Verification items for the finished model (mm, model axes). A direction names the side the tool comes from. Round coordinates to 2 decimals unless told otherwise and drop trailing zeros. Loops run counter-clockwise (first coordinate to the right, second up) from the corner with the lowest first, then second, coordinate; pieces in that order, holes last. Notation, with made-up numbers: M -23.5,-30 L 27.5,-30 A9 ccw 27.5,-13 Z; hole C 82,53.25 d9. An arc over 180 degrees is marked long. One line per item, written item: value.
from build123d import *

# Parameters (mm, degrees)
SALIENTE_EXTRUIR1_DEPTH      = 35
SALIENTE_EXTRUIR1_DEPTH_BACK = 35
CROQUIS3_R                   = 2.5
CORTAR_EXTRUIR1_DEPTH        = 4
CROQUIS4_W                   = 70
CROQUIS4_H                   = 10
CORTAR_EXTRUIR2_DEPTH        = 10


with BuildPart() as part:
    # Croquis2 → Saliente-Extruir1 (new body, two sides)
    with BuildSketch(Plane.XY) as saliente_extruir1_sk:
        Polygon((0, 0), (-50, 0), (-50, -4), (-4, -4), (-4, -50), (0, -50), align=None)
    extrude(amount=SALIENTE_EXTRUIR1_DEPTH)
    extrude(saliente_extruir1_sk.sketch, amount=-SALIENTE_EXTRUIR1_DEPTH_BACK)

    # Croquis3 → Cortar-Extruir1 (cut)
    with BuildSketch(Plane.XZ.offset(4)):
        with Locations((-12, 25)):
            Circle(CROQUIS3_R)
        with Locations((-12, -25)):
            Circle(CROQUIS3_R)
        with Locations((-42, 25)):
            Circle(CROQUIS3_R)
        with Locations((-42, -25)):
            Circle(CROQUIS3_R)
    extrude(amount=-CORTAR_EXTRUIR1_DEPTH, mode=Mode.SUBTRACT)

    # Croquis4 → Cortar-Extruir2 (cut)
    with BuildSketch(Plane.ZY.offset(4)):
        with Locations((0, -45)):
            Rectangle(CROQUIS4_W, CROQUIS4_H)
    extrude(amount=-CORTAR_EXTRUIR2_DEPTH, mode=Mode.SUBTRACT)


solid = part.part
(1) Tool access check on faces 5 (the face through (-4, -22, 0)), 6 (the face through (-25, 0, 0)). Record the directions out of +Z, -Z, +X, -X, +Y, -Y that give a thin tool (end or side, any length) a straight path to the whole face; none if there is none.
Completed:
face 5: +Z, -Z, -X, -Y
face 6: +Z, -Z, +X, -X, +Y
(2) Sectioned sample at D-D on y = -15. Enter the section's corners in (x, z), and give its area (3 significant figures).
Completed:
outline: M -4,-35 L 0,-35 L 0,35 L -4,35 Z
area: 280 mm^2
(3) Mould release check, pull along Z, two halves, no side actions. Record for faces 1 (the face through (-12.33, -2.03, 27.48)), 2 (the face through (-40.66, -2.03, 27.11)), 3 (the face through (-15.9, -3.6, 35)), 4 (the face through (-2, -40, 0)): +Z half, -Z half, draft (parallel to the pull), parting line (faces both ways), or undercut.
Completed:
face 1: undercut
face 2: undercut
face 3: +Z half
face 4: draft
(4) Depth check by flat-ended pin: pin 1 Ø4 at (x, z) = (-42, -25) entering from +Y; pin 2 Ø8 at (x, z) = (-35, 19) entering from -Y; pin 3 Ø18 at (y, z) = (-15, -5) entering from -X. Enter the tip coordinate at first touch or a pass-through.
Completed:
pin 1: passes through
pin 2: stops at y = -4
pin 3: stops at x = -4
(5) Thickness scan on L1, parallel to Z at x = -12, y = -2.2; L2, parallel to Y at x = -11, z = 11. Record the ranges inside material, lowest first. Write a range as from..to.
Completed:
L1: z = -35..-27.5, -22.5..22.5, 27.5..35
L2: y = -4..0
(6) Sectioned sample at B-B on x = -42. Enter the section's corners in (y, z), and give its area (3 significant figures).
Completed:
outline: M -4,-35 L 0,-35 L 0,-27.5 L -4,-27.5 Z; M -4,-22.5 L 0,-22.5 L 0,22.5 L -4,22.5 Z; M -4,27.5 L 0,27.5 L 0,35 L -4,35 Z
area: 240 mm^2
(7) Sectioned sample at A-A on z = 25. Enter the section's corners in (x, y), and give its area (3 significant figures).
Completed:
outline: M -50,-4 L -44.5,-4 L -44.5,0 L -50,0 Z; M -39.5,-4 L -14.5,-4 L -14.5,0 L -39.5,0 Z; M -9.5,-4 L -4,-4 L -4,-40 L 0,-40 L 0,0 L -9.5,0 Z
area: 304 mm^2
(8) Sectioned sample at C-C on z = -3. Enter the section's corners in (x, y).
Completed:
outline: M -50,-4 L -4,-4 L -4,-40 L 0,-40 L 0,0 L -50,0 Z
